Check sheet for the modelled part. Datum: model origin and axes. Units: mm. Give positions to 0.01 mm unless a question says otherwise; leave off trailing zeros. Order: outer loops, then holes, each group sorted by start corner. A loop starts at its lowest first (then second) coordinate and runs counter-clockwise, first axis right, second up. Notation, with made-up numbers: (84, -22) - (94, -22) arc R24 cw to (94, -6) - close; hole circle Ø1 at (42, 34). An arc over 180 degrees is marked (long way). Answer in a Markdown table with one row per item.
from build123d import *

# Parameters (mm, degrees)
SKETCH1_W           = 130
SKETCH1_H           = 92
SKETCH1_R           = 2.3
BOSS_EXTRUDE1_DEPTH = 2
SKETCH2_W           = 58
SKETCH2_H           = 28
BOSS_EXTRUDE2_DEPTH = 4
FILLET1_R           = 10
FILLET2_R           = 2
FILLET3_R           = 0.5
SKETCH3_R           = 8.5
CUT_EXTRUDE1_DEPTH  = 146.86690412


with BuildPart() as part:
    # Sketch1 → Boss-Extrude1 (new body)
    with BuildSketch(Plane(origin=(0, 0, 0), x_dir=(1, 0, 0), z_dir=(0, 1, 0))):
        with Locations((54.9842552, 36.854886379)):
            Rectangle(SKETCH1_W, SKETCH1_H)
        with Locations(Location((0, 74, 0), (0, 0, 270))):
            Circle(SKETCH1_R, mode=Mode.SUBTRACT)
        with Locations(Location((110, 74, 0), (0, 0, 90))):
            Circle(SKETCH1_R, mode=Mode.SUBTRACT)
        with Locations(Location((110, 0, 0), (0, 0, 270))):
            Circle(SKETCH1_R, mode=Mode.SUBTRACT)
        with Locations(Location((0, 0, 0), (0, 0, 90))):
            Circle(SKETCH1_R, mode=Mode.SUBTRACT)
    extrude(amount=BOSS_EXTRUDE1_DEPTH)

    # Sketch2 → Boss-Extrude2 (add)
    with BuildSketch(Plane(origin=(0, 0, 0), x_dir=(1, 0, 0), z_dir=(0, 1, 0))):
        with Locations((54.9842552, 36.854886379)):
            Rectangle(SKETCH2_W, SKETCH2_H)
    extrude(amount=BOSS_EXTRUDE2_DEPTH)

    # Fillet1
    fillet1_edges = [part.edges().sort_by_distance(p)[0] for p in [
        (-10.0157448, 1, -82.854886379),
        (119.9842552, 1, -82.854886379),
        (119.9842552, 1, 9.145113621),
        (-10.0157448, 1, 9.145113621),
    ]]
    fillet(fillet1_edges, radius=FILLET1_R)

    # Fillet2
    fillet2_edges = [part.edges().sort_by_distance(p)[0] for p in [
        (25.9842552, 3, -50.854886379),
        (25.9842552, 3, -22.854886379),
        (83.9842552, 3, -22.854886379),
        (83.9842552, 3, -50.854886379),
    ]]
    fillet(fillet2_edges, radius=FILLET2_R)

    # Fillet3
    fillet3_edges = [part.edges().sort_by_distance(p)[0] for p in [
        (54.9842552, 0, -82.854886379),
        (54.9842552, 2, -82.854886379),
        (-10.0157448, 0, -36.854886379),
        (119.9842552, 0, -36.854886379),
        (54.9842552, 0, 9.145113621),
        (-7.086812612, 0, -79.925954191),
        (-7.086812612, 0, 6.216181433),
        (117.055323011, 0, 6.216181433),
        (117.055323011, 0, -79.925954191),
        (119.9842552, 2, -36.854886379),
        (-10.0157448, 2, -36.854886379),
        (54.9842552, 2, 9.145113621),
        (-7.086812612, 2, -79.925954191),
        (-7.086812612, 2, 6.216181433),
        (117.055323011, 2, 6.216181433),
        (117.055323011, 2, -79.925954191),
        (25.9842552, 4, -36.854886379),
        (54.9842552, 4, -50.854886379),
        (54.9842552, 4, -22.854886379),
        (83.9842552, 4, -36.854886379),
        (26.570041637, 4, -23.440672817),
        (83.398468762, 4, -23.440672817),
        (83.398468762, 4, -50.269099942),
        (26.570041637, 4, -50.269099942),
    ]]
    fillet(fillet3_edges, radius=FILLET3_R)

    # Sketch3 → Cut-Extrude1 (cut, through all)
    with BuildSketch(Plane(origin=(0, 0, 0), x_dir=(1, 0, 0), z_dir=(0, 1, 0))):
        with Locations(Location((54.9842552, 36.854886379, 0), (0, 0, 270))):
            Circle(SKETCH3_R)
    extrude(amount=CUT_EXTRUDE1_DEPTH, mode=Mode.SUBTRACT)


solid = part.part
(1) Cross-section at C-C, the plane x = 52.5. Record the cut outline in (y, z), then the cut area to 3 significant figures.
Geometry says:
| item | result |
|---|---|
| outline | (0, -82.35) arc R0.5 ccw to (0.5, -82.85) - (1.5, -82.85) arc R0.5 ccw to (2, -82.35) - (2, -50.85) - (3.5, -50.85) arc R0.5 ccw to (4, -50.35) - (4, -44.98) - (0, -44.98) - close; (0, -28.73) - (4, -28.73) - (4, -23.35) arc R0.5 ccw to (3.5, -22.85) - (2, -22.85) - (2, 8.65) arc R0.5 ccw to (1.5, 9.15) - (0.5, 9.15) arc R0.5 ccw to (0, 8.65) - close |
| area | 175 mm² |
(2) Cross-section at B-B, the plane x = 68. Record the cut outline in (y, z).
Geometry says:
| item | result |
|---|---|
| outline | (0, -82.35) arc R0.5 ccw to (0.5, -82.85) - (1.5, -82.85) arc R0.5 ccw to (2, -82.35) - (2, -50.85) - (3.5, -50.85) arc R0.5 ccw to (4, -50.35) - (4, -23.35) arc R0.5 ccw to (3.5, -22.85) - (2, -22.85) - (2, 8.65) arc R0.5 ccw to (1.5, 9.15) - (0.5, 9.15) arc R0.5 ccw to (0, 8.65) - close |
(3) Mould release check, pull along Z, two halves, no side actions. Record for faces 1 (the cylindrical face through (-0.881, 0.986, -71.875)), 2 (the cylindrical face through (60.73, 1.97, -43.12)), 3 (the cylindrical face through (-7.2, 1, 6.1)), 4 (the flat face through (54, 2, -58)): pulls with the +Z half, pulls with the -Z half, needs draft (parallel to the pull), parting line crosses it, or undercut.
Geometry says:
| item | result |
|---|---|
| face 1 | undercut |
| face 2 | undercut |
| face 3 | pulls with the +Z half |
| face 4 | needs draft |
(4) Thickness scan on L1, parallel to Z at x = 1.5, y = 1.4; L2, parallel to Z at x = 103, y = 0.4; L3, parallel to X at y = 0.75, z = -74. Record the ranges inside material, lowest first.
Geometry says:
| item | result |
|---|---|
| L1 | -82.85 to -75.74, -72.26 to -1.74, 1.74 to 9.15 |
| L2 | -82.84 to 9.14 |
| L3 | -9.95 to -2.3, 2.3 to 107.7, 112.3 to 119.92 |
(5) Gauge pin test, flat ends, axial feed: P1, Ø6, axis at x = 0, z = 0, coming from the -Y side; P2, Ø1.2, axis at y = 3, z = -36.5, coming from the +X side; P3, Ø7.5, axis at x = 110, z = -74, coming from the +Y side; P4, Ø10, axis at x = 54.98, z = -36.85, coming from the -Y side. Record the tip position at first contact, or that the pin passes through.
Geometry says:
| item | result |
|---|---|
| P1 | y = 0 |
| P2 | x = 83.98 |
| P3 | y = 2 |
| P4 | through |
(6) Cross-section at A-A, the plane z = -66.5. Record the cut outline in (x, y), then the cut area to 3 significant figures.
Geometry says:
| item | result |
|---|---|
| outline | (-10.02, 0.5) arc R0.5 ccw to (-9.52, 0) - (119.48, 0) arc R0.5 ccw to (119.98, 0.5) - (119.98, 1.5) arc R0.5 ccw to (119.48, 2) - (-9.52, 2) arc R0.5 ccw to (-10.02, 1.5) - close |
| area | 260 mm² |
(7) Cross-section at D-D, the plane x = 7. Record the cut outline in (y, z).
Geometry says:
| item | result |
|---|---|
| outline | (0, -82.35) arc R0.5 ccw to (0.5, -82.85) - (1.5, -82.85) arc R0.5 ccw to (2, -82.35) - (2, 8.65) arc R0.5 ccw to (1.5, 9.15) - (0.5, 9.15) arc R0.5 ccw to (0, 8.65) - close |
